Read the model definition and answer for the solid it produces. Units are mm, in the model's axes. A direction names the side the tool comes from. Coordinates: 2 decimals unless noted, no trailing zeros. Write each loop counter-clockwise with the first axis right and the second up, starting at its lowest first coordinate (ties: lowest second). Pieces come first, ordered by that corner, then holes.
Item 1: A tool of negligible diameter and unlimited length cuts with its end or side. For faces 4 (the face through (-3, -300, 147)), 5 (the face through (3, 4, -1)), from which of +Z, -Z, +X, -X, +Y, -Y can it reach the whole face along a straight path? Write none if from no direction.
Item 2: Section C-C (y = 18) is taken. Give the vertices of the cut face in (x, z).
Item 3: Determine the mould class of faces 1 (the face through (201, -4, 151)), 2 (the face through (3, -301, 151)), 3 (the face through (3, 4, 0)) for opening direction Y: released by +Y, released by -Y, zero draft, split by the parting line, or undercut.
Item 4: Section B-B (x = -51) is taken. Give the vertices of the cut face in (y, z).
Item 5: This flat-tipped pin is pushed along its axis until it touches: P1, Ø2, axis at x = -147.5, y = 107.5, coming from the +Z side. Where does it stop, or does it pass through?
Item 6: Straight lines are drawn through the part: probe 1 along X at (y, z) = (153, 55); probe 2 along Y at (x, z) = (-3.5, 209); probe 3 along Z at (x, y) = (-102, -66.5). For each, find the intervals that lie inside material, in ascending order.
Item 7: Section A-A (z = 50) is taken. Give the vertices of the cut face in (x, y).
from build123d import *

# Parameters (mm, degrees)
SKETCH1_W           = 402
SKETCH1_H           = 602
SKETCH1_W_2         = 400
SKETCH1_H_2         = 600
BOSS_EXTRUDE1_DEPTH = 299
SKETCH2_W           = 402
SKETCH2_H           = 602
BOSS_EXTRUDE2_DEPTH = 1


with BuildPart() as part:
    # Sketch1 → Boss-Extrude1 (new body)
    with BuildSketch(Plane.XY):
        Rectangle(SKETCH1_W, SKETCH1_H)
        Rectangle(SKETCH1_W_2, SKETCH1_H_2, mode=Mode.SUBTRACT)
    extrude(amount=BOSS_EXTRUDE1_DEPTH)

    # Sketch2 → Boss-Extrude2 (add)
    with BuildSketch(Plane(origin=(0, 0, 0), x_dir=(-1, 0, 0), z_dir=(0, 0, -1))):
        Rectangle(SKETCH2_W, SKETCH2_H)
    extrude(amount=BOSS_EXTRUDE2_DEPTH)


solid = part.part
Established:
1. face 4: +Z
1. face 5: -Z, +X, -X, +Y, -Y
2. outline: (-201, -1) - (201, -1) - (201, 299) - (200, 299) - (200, 0) - (-200, 0) - (-200, 299) - (-201, 299) - close
3. face 1: zero draft
3. face 2: released by -Y
3. face 3: undercut
4. outline: (-301, -1) - (301, -1) - (301, 299) - (300, 299) - (300, 0) - (-300, 0) - (-300, 299) - (-301, 299) - close
5. P1: stops at z = 0
6. probe 1: x = -201 to -200, 200 to 201
6. probe 2: y = -301 to -300, 300 to 301
6. probe 3: z = -1 to 0
7. outline: (-201, -301) - (201, -301) - (201, 301) - (-201, 301) - close; hole (-200, -300) - (200, -300) - (200, 300) - (-200, 300) - close
